Check sheet for the drawn part. Datum: minimum x, y, z corner. Units: mm. A direction names the side the tool comes from. Give positions to 0.01 mm unless a question says otherwise; leave off trailing zeros. Write each loop counter-clockwise with the first axis right and the second up, starting at its lowest first coordinate (ties: lowest second). Pieces come first, ordered by that corner, then holes. Notation, with made-up numbers: M 6,39 L 22,39 A24 ccw 22,68 Z; hole C 88,-18.5 d4. An arc over 180 degrees is marked long. Write item = value, one per line.
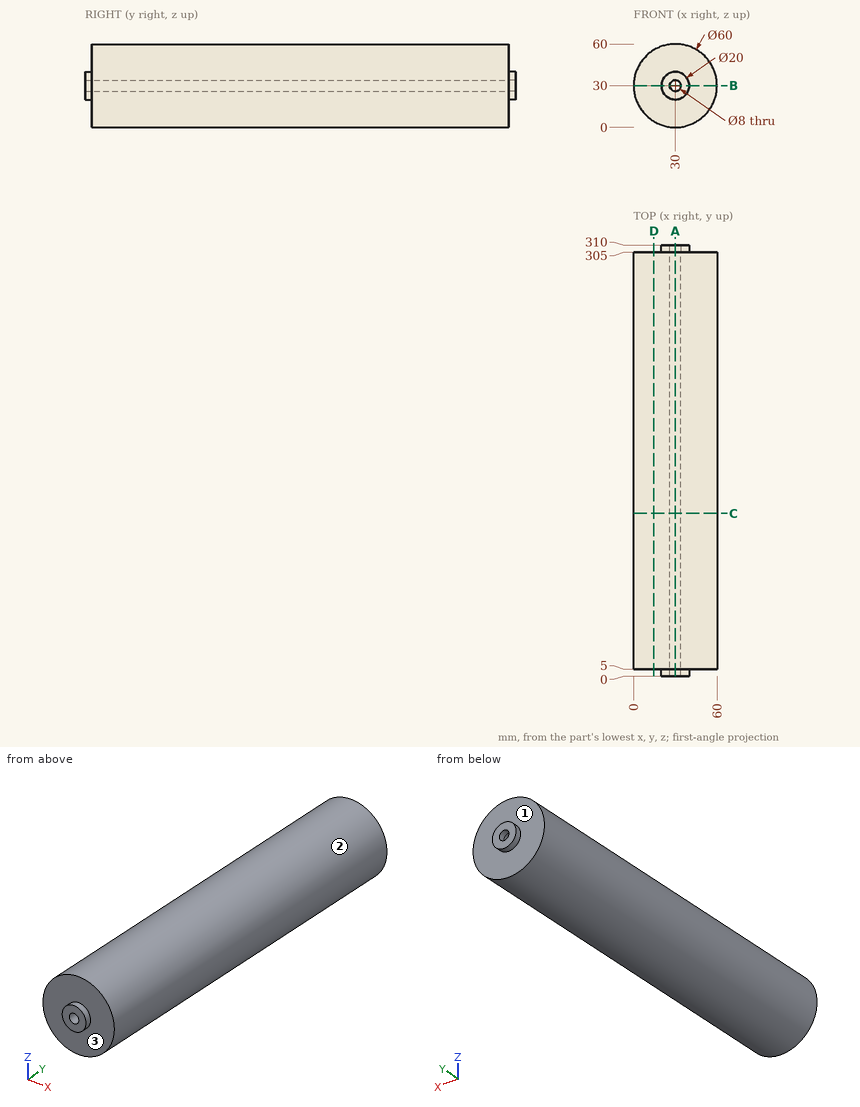
1) Cross-section at D-D on x = 14.5. Record the boundary of the cut face in (y, z), plus the area to 3 significant figures.
From the geometry:
outline = M 5,4.31 L 305,4.31 L 305,55.69 L 5,55.69 Z
area = 15,400 mm^2
2) Depth check by flat-ended pin: P1, Ø12, axis at x = 12, z = 32, coming from the -Y side; P2, Ø5, axis at y = 108, z = 38, coming from the +X side; P3, Ø3, axis at y = 55, z = 14.5, coming from the +X side; P4, Ø7, axis at x = 30, z = 30, coming from the +Y side. Enter the tip coordinate at first touch or a pass-through.
From the geometry:
P1 = 5
P2 = 59.49
P3 = 56.53
P4 = through
3) Cross-section at A-A on x = 30. Record the boundary of the cut face in (y, z), plus the area to 3 significant figures.
From the geometry:
outline = M 0,20 L 5,20 L 5,0 L 305,0 L 305,20 L 310,20 L 310,26 L 0,26 Z; M 0,34 L 310,34 L 310,40 L 305,40 L 305,60 L 5,60 L 5,40 L 0,40 Z
area = 15,700 mm^2
4) Cross-section at C-C on y = 117. Record the boundary of the cut face in (x, z).
From the geometry:
outline = C 30,30 d60; hole C 30,30 d8
5) Cross-section at B-B on z = 30. Record the boundary of the cut face in (x, y), plus the area to 3 significant figures.
From the geometry:
outline = M 0,5 L 20,5 L 20,0 L 26,0 L 26,310 L 20,310 L 20,305 L 0,305 Z; M 34,0 L 40,0 L 40,5 L 60,5 L 60,305 L 40,305 L 40,310 L 34,310 Z
area = 15,700 mm^2
6) Tool access check on the marked faces 1, 2 and 3. Record the directions out of +Z, -Z, +X, -X, +Y, -Y that give a thin tool (end or side, any length) a straight path to the whole face; none if there is none.
From the geometry:
face_1 = +Y
face_2 = +Y, -Y
face_3 = -Y
7) Material ranges on probe 1 along Z at (x, y) = (30, 306.05); probe 2 along Z at (x, y) = (30, 194); probe 3 along Y at (x, z) = (38, 41), recorded low to high. Write a range as from..to.
From the geometry:
probe_1 = 20..26, 34..40
probe_2 = 0..26, 34..60
probe_3 = 5..305
